Could you check a few things on this model? Use its own coordinates, in mm. Face numbers are marked on the shaded views. A direction names the side the tool comes from. Coordinates: 2 decimals unless noted, no trailing zeros. Loops run counter-clockwise (first coordinate to the right, second up) from the corner with the lowest first, then second, coordinate; pieces in that order, holes last. Notation, with made-up numbers: M -6.75,27.25 L 22.25,27.25 A37 ccw 22.25,66.25 Z; hole C -6,71 d11. An arc over 180 degrees is marked long. Return JSON: item names as keys, results as strings. Group by question number.
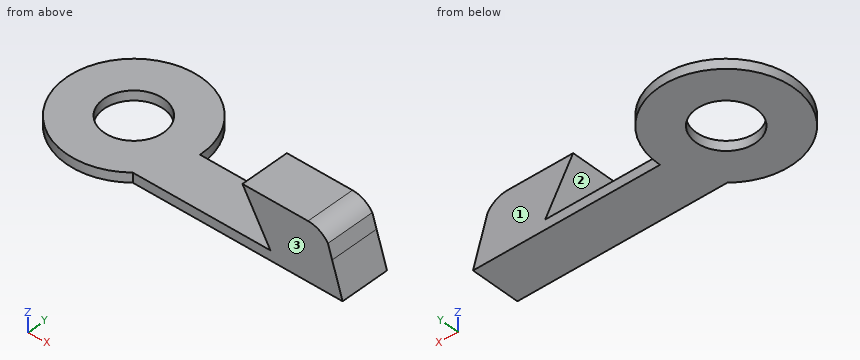
from build123d import *

# Parameters (mm, degrees)
BOSS_EXTRUDE1_DEPTH     = 5.1
SKETCH4_W               = 1
SKETCH4_H               = 5.1
BOSS_EXTRUDE2_DEPTH     = 18.9
SKETCH5_R               = 7
BOSS_EXTRUDE3_DEPTH     = 1
CUT_EXTRUDE1_DEPTH      = 33.605252644
CUT_EXTRUDE1_DEPTH_BACK = 33.605252644
SKETCH6_R               = 3.1
BOSS_EXTRUDE4_DEPTH     = 5.1
CUT_EXTRUDE2_DEPTH      = 10
BOSS_EXTRUDE5_DEPTH     = 5.1


with BuildPart() as part:
    # Sketch3 → Boss-Extrude1 (new body)
    with BuildSketch(Plane(origin=(0, 0, 0), x_dir=(1, 0, 0), z_dir=(0, 1, 0))):
        with BuildLine():
            Line((0, -2.5), (-3.9, -2.5))
            Line((-3.9, -2.5), (-3.9, 3.5))
            Line((-3.9, 3.5), (-1, 3.5))
            ThreePointArc((-1, 3.5), (1.474873734, 2.474873734), (2.5, 0))
            ThreePointArc((2.5, 0), (1.767766953, -1.767766953), (0, -2.5))
        make_face()
    extrude(amount=BOSS_EXTRUDE1_DEPTH)

    # Sketch4 → Boss-Extrude2 (add)
    with BuildSketch(Plane.ZY.offset(3.9)):
        with Locations((-3, 2.55)):
            Rectangle(SKETCH4_W, SKETCH4_H)
    extrude(amount=BOSS_EXTRUDE2_DEPTH)

    # Sketch5 → Boss-Extrude3 (add)
    with BuildSketch(Plane(origin=(0, 0, -3.5), x_dir=(-1, 0, 0), z_dir=(0, 0, -1))):
        with Locations((22.8, 5.25)):
            Circle(SKETCH5_R)
    extrude(amount=-BOSS_EXTRUDE3_DEPTH)

    # Sketch6 → Cut-Extrude1 (cut, two sides: drawn at the far end of the back side and taken through both)
    with BuildSketch(Plane.XY.offset(-2.5).offset(-CUT_EXTRUDE1_DEPTH_BACK)):
        with Locations((-22.8, 5.25)):
            Circle(SKETCH6_R)
    extrude(amount=CUT_EXTRUDE1_DEPTH + CUT_EXTRUDE1_DEPTH_BACK, mode=Mode.SUBTRACT)

    # Sketch7 → Boss-Extrude4 (add)
    with BuildSketch(Plane.XZ):
        Polygon((-3.9, -2.5), (-3.9, 2.5), (-6.8, 2.5), align=None)
    extrude(amount=-BOSS_EXTRUDE4_DEPTH)

    # Sketch8 → Cut-Extrude2 (cut)
    with BuildSketch(Plane(origin=(0, 5.1, 0), x_dir=(1, 0, 0), z_dir=(0, 1, 0))):
        Polygon((2.5, 0), (0.957021589, -5), (5.957021589, -5), (5.957021589, 0), align=None)
    extrude(amount=-CUT_EXTRUDE2_DEPTH, mode=Mode.SUBTRACT)

    # Sketch9 → Boss-Extrude5 (add)
    with BuildSketch(Plane(origin=(0, 0, 0), x_dir=(1, 0, 0), z_dir=(0, 1, 0))):
        Polygon((2.5, 0), (3.580084888, 3.5), (-1, 3.5), align=None)
    extrude(amount=BOSS_EXTRUDE5_DEPTH)


solid = part.part
(1) Imagine slicing it at D-D, the plane x = 1.5. Write out the boundary of the cut face in (y, z), then the cut area to 4 significant figures.
(2) Imagine slicing it at B-B, the plane y = 2.75. Write out the boundary of the cut face in (x, z).
(3) Imagine slicing it at A-A, the plane x = -22.8. Write out the boundary of the cut face in (y, z), then the cut area to 3 significant figures.
(4) If I drill on L1, parallel to X at y = 5.25, z = -3.2; L2, parallel to Y at x = -22.8, z = -2.8; L3, parallel to Z at x = -17, y = 3, over which ranges is the centre line in solid material (lowest first)? Write a range as [from, to].
(5) For the marked faces 1, 2 and 3, which set-ups out of +Z, -Z, +X, -X, +Y, -Y let a thin tool reach every point of the face, with its end or its side?
(6) Imagine slicing it at C-C, the plane z = 2. Write out the boundary of the cut face in (x, y).
(7) Will this pin go through, and if not, where does the flat tip stop? P1, Ø1, axis at x = -23, y = 8.5, coming from the +Z side.
Checks:
{
 "1": {"outline": "M 0,-3.5 L 5.1,-3.5 L 5.1,2 L 0,2 Z", "area": "28.05 mm²"},
 "2": {"outline": "M -29.34,-3.5 L -24.63,-3.5 L -24.63,-2.5 L -29.34,-2.5 Z; M -20.97,-3.5 L 3.58,-3.5 L 2.07,1.41 A2.5 ccw 0,2.5 L -6.8,2.5 L -3.9,-2.5 L -20.97,-2.5 Z"},
 "3": {"outline": "M -1.75,-3.5 L 2.15,-3.5 L 2.15,-2.5 L -1.75,-2.5 Z; M 8.35,-3.5 L 12.25,-3.5 L 12.25,-2.5 L 8.35,-2.5 Z", "area": "7.80 mm²"},
 "4": {"L1": "[-29.8, -25.9], [-19.7, -15.8]", "L2": "[-1.75, 2.15], [8.35, 12.25]", "L3": "[-3.5, -2.5]"},
 "5": {"face 1": "+Z, -Z, +X, +Y", "face 2": "-X, +Y, -Y", "face 3": "+Z, -Z, +X, -Y"},
 "6": {"outline": "M -6.51,0 L 1.5,0 L 1.5,5.1 L -6.51,5.1 Z"},
 "7": {"P1": "z = -2.5"}
}
